from build123d import *

# Parameters (mm, degrees)
SKETCH1_R           = 280
BOSS_EXTRUDE1_DEPTH = 50
SKETCH2_R           = 250
BOSS_EXTRUDE2_DEPTH = 10
SKETCH3_R           = 120
BOSS_EXTRUDE3_DEPTH = 150
DRAFT1_ANGLE        = 10
SKETCH4_R           = 260
BOSS_EXTRUDE4_DEPTH = 600
CUT_EXTRUDE1_START  = -600
CUT_EXTRUDE1_DEPTH  = 600
SKETCH6_R           = 225
BOSS_EXTRUDE5_DEPTH = 600
SKETCH7_R           = 260
BOSS_EXTRUDE6_DEPTH = 60
SKETCH9_R           = 160


with BuildPart() as part:
    # Sketch1 → Boss-Extrude1 (new body)
    with BuildSketch(Plane(origin=(0, 0, 0), x_dir=(0, 0, -1), z_dir=(1, 0, 0))):
        Circle(SKETCH1_R)
    extrude(amount=BOSS_EXTRUDE1_DEPTH)

    # Sketch2 → Boss-Extrude2 (add)
    with BuildSketch(Plane(origin=(50, 0, 0), x_dir=(0, 0, -1), z_dir=(1, 0, 0))):
        Circle(SKETCH2_R)
    extrude(amount=BOSS_EXTRUDE2_DEPTH)

    # Sketch3 → Boss-Extrude3 (add)
    with BuildSketch(Plane(origin=(60, 0, 0), x_dir=(0, 0, -1), z_dir=(1, 0, 0))):
        Circle(SKETCH3_R)
    extrude(amount=BOSS_EXTRUDE3_DEPTH)

    # Draft1
    draft1_faces = [part.faces().sort_by_distance(p)[0] for p in [
        (135, 0, 120),
    ]]
    draft(draft1_faces, Plane(origin=(210, 0, 0), x_dir=(0, 0, 1), z_dir=(1, 0, 0)), DRAFT1_ANGLE)

    # Sketch4 → Boss-Extrude4 (add)
    with BuildSketch(Plane.ZY):
        Circle(SKETCH4_R)
    extrude(amount=BOSS_EXTRUDE4_DEPTH)

    # Sketch5 → Cut-Extrude1 (cut)
    with BuildSketch(Plane.ZY.offset(600).offset(CUT_EXTRUDE1_START)):
        with BuildLine():
            Line((87.550166574, 244.816192955), (46.587428118, 173.866648732))
            Line((46.587428118, 173.866648732), (46.587428118, 255.792125644))
            ThreePointArc((46.587428118, 255.792125644), (67.292951727, 251.140714835), (87.550166574, 244.816192955))
        make_face()
        with BuildLine():
            Line((21.203873704, 259.13393398), (0, 180))
            Line((0, 180), (-21.203873704, 259.13393398))
            ThreePointArc((-21.203873704, 259.13393398), (0, 260), (21.203873704, 259.13393398))
        make_face()
        with BuildLine():
            Line((147.930060276, 213.814632957), (90, 155.884572681))
            Line((90, 155.884572681), (111.203873704, 235.018506661))
            ThreePointArc((111.203873704, 235.018506661), (130, 225.166604984), (147.930060276, 213.814632957))
        make_face()
        with BuildLine():
            Line((198.228764836, 168.241959069), (127.279220614, 127.279220614))
            Line((127.279220614, 127.279220614), (168.241959069, 198.228764836))
            ThreePointArc((168.241959069, 198.228764836), (183.847763109, 183.847763109), (198.228764836, 168.241959069))
        make_face()
        with BuildLine():
            Line((235.018506661, 111.203873704), (155.884572681, 90))
            Line((155.884572681, 90), (213.814632957, 147.930060276))
            ThreePointArc((213.814632957, 147.930060276), (225.166604984, 130), (235.018506661, 111.203873704))
        make_face()
        with BuildLine():
            Line((255.792125644, 46.587428118), (173.866648732, 46.587428118))
            Line((173.866648732, 46.587428118), (244.816192955, 87.550166574))
            ThreePointArc((244.816192955, 87.550166574), (251.140714835, 67.292951727), (255.792125644, 46.587428118))
        make_face()
        with BuildLine():
            Line((259.13393398, -21.203873704), (180, 0))
            Line((180, 0), (259.13393398, 21.203873704))
            ThreePointArc((259.13393398, 21.203873704), (260, 0), (259.13393398, -21.203873704))
        make_face()
        with BuildLine():
            Line((244.816192955, -87.550166574), (173.866648732, -46.587428118))
            Line((173.866648732, -46.587428118), (255.792125644, -46.587428118))
            ThreePointArc((255.792125644, -46.587428118), (251.140714835, -67.292951727), (244.816192955, -87.550166574))
        make_face()
        with BuildLine():
            Line((213.814632957, -147.930060276), (155.884572681, -90))
            Line((155.884572681, -90), (235.018506661, -111.203873704))
            ThreePointArc((235.018506661, -111.203873704), (225.166604984, -130), (213.814632957, -147.930060276))
        make_face()
        with BuildLine():
            Line((168.241959069, -198.228764836), (127.279220614, -127.279220614))
            Line((127.279220614, -127.279220614), (198.228764836, -168.241959069))
            ThreePointArc((198.228764836, -168.241959069), (183.847763109, -183.847763109), (168.241959069, -198.228764836))
        make_face()
        with BuildLine():
            Line((111.203873704, -235.018506661), (90, -155.884572681))
            Line((90, -155.884572681), (147.930060276, -213.814632957))
            ThreePointArc((147.930060276, -213.814632957), (130, -225.166604984), (111.203873704, -235.018506661))
        make_face()
        with BuildLine():
            Line((46.587428118, -255.792125644), (46.587428118, -173.866648732))
            Line((46.587428118, -173.866648732), (87.550166574, -244.816192955))
            ThreePointArc((87.550166574, -244.816192955), (67.292951727, -251.140714835), (46.587428118, -255.792125644))
        make_face()
        with BuildLine():
            Line((-21.203873704, -259.13393398), (0, -180))
            Line((0, -180), (21.203873704, -259.13393398))
            ThreePointArc((21.203873704, -259.13393398), (0, -260), (-21.203873704, -259.13393398))
        make_face()
        with BuildLine():
            Line((-87.550166574, -244.816192955), (-46.587428118, -173.866648732))
            Line((-46.587428118, -173.866648732), (-46.587428118, -255.792125644))
            ThreePointArc((-46.587428118, -255.792125644), (-67.292951727, -251.140714835), (-87.550166574, -244.816192955))
        make_face()
        with BuildLine():
            Line((-147.930060276, -213.814632957), (-90, -155.884572681))
            Line((-90, -155.884572681), (-111.203873704, -235.018506661))
            ThreePointArc((-111.203873704, -235.018506661), (-130, -225.166604984), (-147.930060276, -213.814632957))
        make_face()
        with BuildLine():
            Line((-198.228764836, -168.241959069), (-127.279220614, -127.279220614))
            Line((-127.279220614, -127.279220614), (-168.241959069, -198.228764836))
            ThreePointArc((-168.241959069, -198.228764836), (-183.847763109, -183.847763109), (-198.228764836, -168.241959069))
        make_face()
        with BuildLine():
            Line((-235.018506661, -111.203873704), (-155.884572681, -90))
            Line((-155.884572681, -90), (-213.814632957, -147.930060276))
            ThreePointArc((-213.814632957, -147.930060276), (-225.166604984, -130), (-235.018506661, -111.203873704))
        make_face()
        with BuildLine():
            Line((-255.792125644, -46.587428118), (-173.866648732, -46.587428118))
            Line((-173.866648732, -46.587428118), (-244.816192955, -87.550166574))
            ThreePointArc((-244.816192955, -87.550166574), (-251.140714835, -67.292951727), (-255.792125644, -46.587428118))
        make_face()
        with BuildLine():
            Line((-259.13393398, 21.203873704), (-180, 0))
            Line((-180, 0), (-259.13393398, -21.203873704))
            ThreePointArc((-259.13393398, -21.203873704), (-260, 0), (-259.13393398, 21.203873704))
        make_face()
        with BuildLine():
            Line((-244.816192955, 87.550166574), (-173.866648732, 46.587428118))
            Line((-173.866648732, 46.587428118), (-255.792125644, 46.587428118))
            ThreePointArc((-255.792125644, 46.587428118), (-251.140714835, 67.292951727), (-244.816192955, 87.550166574))
        make_face()
        with BuildLine():
            Line((-213.814632957, 147.930060276), (-155.884572681, 90))
            Line((-155.884572681, 90), (-235.018506661, 111.203873704))
            ThreePointArc((-235.018506661, 111.203873704), (-225.166604984, 130), (-213.814632957, 147.930060276))
        make_face()
        with BuildLine():
            Line((-168.241959069, 198.228764836), (-127.279220614, 127.279220614))
            Line((-127.279220614, 127.279220614), (-198.228764836, 168.241959069))
            ThreePointArc((-198.228764836, 168.241959069), (-183.847763109, 183.847763109), (-168.241959069, 198.228764836))
        make_face()
        with BuildLine():
            Line((-111.203873704, 235.018506661), (-90, 155.884572681))
            Line((-90, 155.884572681), (-147.930060276, 213.814632957))
            ThreePointArc((-147.930060276, 213.814632957), (-130, 225.166604984), (-111.203873704, 235.018506661))
        make_face()
        with BuildLine():
            Line((-46.587428118, 255.792125644), (-46.587428118, 173.866648732))
            Line((-46.587428118, 173.866648732), (-87.550166574, 244.816192955))
            ThreePointArc((-87.550166574, 244.816192955), (-67.292951727, 251.140714835), (-46.587428118, 255.792125644))
        make_face()
    extrude(amount=CUT_EXTRUDE1_DEPTH, mode=Mode.SUBTRACT)

    # Sketch6 → Boss-Extrude5 (add)
    with BuildSketch(Plane.ZY.offset(600)):
        Circle(SKETCH6_R)
    extrude(amount=-BOSS_EXTRUDE5_DEPTH)

    # Sketch7 → Boss-Extrude6 (add)
    with BuildSketch(Plane.ZY.offset(600)):
        with Locations(Location((0, 0, 0), (0, 0, 184.677858529))):
            Circle(SKETCH7_R)
    extrude(amount=BOSS_EXTRUDE6_DEPTH)

    # Sketch9 → section 1 of loft1
    with BuildSketch(Plane.ZY.offset(810), mode=Mode.PRIVATE) as loft1_s1:
        Circle(SKETCH9_R)
    # loft from a face of the part (loft1)
    loft([part.faces().sort_by_distance((-660, 0, 0))[0], loft1_s1.sketch])


solid = part.part
Input: part model. Units: mm. Frame: model coordinates. A direction names the side the tool comes from. Coordinates: 2 decimals unless noted, no trailing zeros. Loops run counter-clockwise (first coordinate to the right, second up) from the corner with the lowest first, then second, coordinate; pieces in that order, holes last. Notation, with made-up numbers: (63.25, 25) - (112.25, 25) arc R32 cw to (112.25, 61) - close; hole circle Ø3 at (59, 35). An arc over 180 degrees is marked (long way). Answer in a Markdown table with one row per item. Add a question column.
Item 1: Contact query for flat-ended pins moving along their axis: P1, Ø8, axis at x = -389.5, z = -150, coming from the -Y side; P2, Ø10.5, axis at x = -388, y = 245, coming from the +Z side; P3, Ø24, axis at y = -172.5, z = 172.5, coming from the +X side. Output: stop coordinate, or through.
Item 2: Access query for faces 1 (the flat face through (-295.8, -135.143, -201.028)), 2 (the flat face through (-295.8, 241.666, -16.523)), 3 (the flat face through (-295.8, 106.65, 218.03)), 4 (the flat face through (50, 229, 105)). Directions: +Z, -Z, +X, -X, +Y, -Y. A direction counts if a zero-diameter tool reaches every point of the face in a straight line with its end or side. Return the directions, or none.
Item 3: Mould query, pull axis Z, two halves, no side actions, for faces 5 (the flat face through (-296, -46.587, -238)), 6 (the flat face through (-296, 238, -46.587)), 7 (the flat face through (-295.8, 78.51, 229.16)). Classes: released by +Z, released by -Z, zero draft, split by the parting line, or undercut.
Item 4: Section query A-A on y = 0. Return the cut outline in (x, z).
Item 5: Line query: line 1 along Y through (x, z) = (-210.5, -211); line 2 along Z through (x, y) = (-4, 9); line 3 along Z through (x, y) = (-526, 253). Output: solid intervals per line, ascending. Write a range as [from, to].
Recorded:
| question | item | result |
|---|---|---|
| 1 | P1 | y = -213.81 |
| 1 | P2 | z = 100.6 |
| 1 | P3 | x = 60 |
| 2 | face 1 | -Z |
| 2 | face 2 | +Y |
| 2 | face 3 | none |
| 2 | face 4 | +X |
| 3 | face 5 | zero draft |
| 3 | face 6 | undercut |
| 3 | face 7 | released by +Z |
| 4 | outline | (-810, -160) - (-660, -260) - (-600, -260) - (-600, -225) - (0, -225) - (0, -280) - (50, -280) - (50, -250) - (60, -250) - (60, -146.45) - (210, -120) - (210, 120) - (60, 146.45) - (60, 250) - (50, 250) - (50, 280) - (0, 280) - (0, 225) - (-600, 225) - (-600, 260) - (-660, 260) - (-810, 160) - close |
| 5 | line 1 | [-151.92, -145.12], [-104.77, 104.77], [145.12, 151.92] |
| 5 | line 2 | [-224.82, 224.82] |
| 5 | line 3 | [-46.59, -19.56], [19.56, 46.59] |
